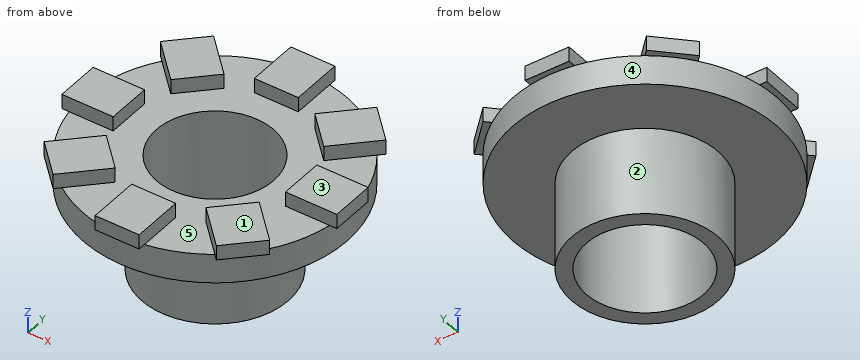
```python
from build123d import *

# Parameters (mm, degrees)
F4_DEPTH = 6.35
F5_COUNT = 8


# Not quite as in the source:
# - a feature names something its author has since deleted; it is built from what else it names


with BuildPart() as f1:
    # F0 (on Front) → F1 (revolve)
    with BuildSketch(Plane.XZ):
        Polygon((25.4, 0), (25.4, -50.8), (31.75, -50.8), (31.75, -12.7), (57.15, -12.7), (57.15, 0), align=None)
    revolve(axis=Axis((0, 0, 2.673143521), (0, 0, -1)))

    # F2 (on face) → F4 (join)
    with BuildSketch(Plane.XY):
        with BuildLine():
            ThreePointArc((57.15, 0), (56.9498143774, -4.779240775), (56.350659934, -9.525))
            Line((56.350659934, -9.525), (59.525659934, -9.525))
            Line((59.525659934, -9.525), (59.525659934, 9.525))
            Line((59.525659934, 9.525), (56.350659934, 9.525))
            ThreePointArc((56.350659934, 9.525), (56.9498143774, 4.779240775), (57.15, 0))
        make_face()
        with BuildLine():
            Line((37.300659934, 9.525), (37.300659934, -9.525))
            Line((37.300659934, -9.525), (56.350659934, -9.525))
            ThreePointArc((56.350659934, -9.525), (56.9498143774, -4.779240775), (57.15, 0))
            ThreePointArc((57.15, 0), (56.9498143774, 4.779240775), (56.350659934, 9.525))
            Line((56.350659934, 9.525), (37.300659934, 9.525))
        make_face()
    extrude(amount=F4_DEPTH)

    # F5: F1 ×8 about axis
    f5_axis = Axis((0, 0, 22.2758), (0, 0, 1))


with BuildPart() as f1_1:
    add(f1.part)
    for i in range(1, F5_COUNT):
        add(f1.part.rotate(f5_axis, i * 360 / F5_COUNT))


solid = f1_1.part
```
Work out the finished part from the listing and answer in its coordinate system (mm). Face numbers are marked on the shaded views. A direction names the side the tool comes from. Round coordinates to 2 decimals unless told otherwise and drop trailing zeros. Loops run counter-clockwise (first coordinate to the right, second up) from the corner with the lowest first, then second, coordinate; pieces in that order, holes last.
(1) The part is cut by section D-D, the plane x = -28.5. Give the vertices of the cut face in (y, z).
Computed values:
outline: (-49.54, -12.7) - (-13.99, -12.7) - (-13.99, -50.8) - (13.99, -50.8) - (13.99, -12.7) - (49.54, -12.7) - (49.54, 0) - (41.97, 0) - (41.97, 6.35) - (24.25, 6.35) - (24.25, 0) - (-24.25, 0) - (-24.25, 6.35) - (-41.97, 6.35) - (-41.97, 0) - (-49.54, 0) - close
(2) For the marked faces 1 and 2, determine the directions among +Z, -Z, +X, -X, +Y, -Y from which every point of the face is accessible in a straight line to the end or side of a thin tool.
Computed values:
face 1: +Z, +X, -X, +Y, -Y
face 2: -Z
(3) Find the intervals of material crossed by L1, parallel to Y at x = 0, z = -39; L2, parallel to Z at x = 41, y = 28, in increasing order.
Computed values:
L1: y = -31.75 to -25.4, 25.4 to 31.75
L2: z = -12.7 to 6.35
(4) The part is cut by section A-A, the plane x = 0. Give the vertices of the cut face in (y, z), and give its area (3 significant figures).
Computed values:
outline: (-59.53, 0) - (-57.15, 0) - (-57.15, -12.7) - (-31.75, -12.7) - (-31.75, -50.8) - (-25.4, -50.8) - (-25.4, 0) - (-37.3, 0) - (-37.3, 6.35) - (-59.53, 6.35) - close; (25.4, -50.8) - (31.75, -50.8) - (31.75, -12.7) - (57.15, -12.7) - (57.15, 0) - (59.53, 0) - (59.53, 6.35) - (37.3, 6.35) - (37.3, 0) - (25.4, 0) - close
area: 1,570 mm2
(5) Each of these flat-tipped pins is pushed along its axis until it touches: P1, Ø4, axis at y = 19.5, z = -12.5, coming from the -X side; P2, Ø1.6, axis at x = 58.5, y = -2, coming from the -Z side; P3, Ø7, axis at x = -54, z = 4.5, coming from the +Y side (3 decimals); P4, Ø6, axis at y = 47, z = -18.5, coming from the +X side. Where does it stop, or does it pass through?
Computed values:
P1: stops at x = -54.4
P2: stops at z = 0
P3: stops at y = 9.525
P4: passes through
(6) The mould has two halves that part along X. Classify the marked faces 3, 4 and 5: pulls with the +X half, pulls with the -X half, needs draft (parallel to the pull), parting line crosses it, or undercut.
Computed values:
face 3: needs draft
face 4: parting line crosses it
face 5: undercut
(7) The part is cut by section C-C, the plane z = -17.5. Give the vertices of the cut face in (x, y), and give its area (3 significant figures).
Computed values:
outline: circle Ø63.5 at (0, 0); hole circle Ø50.8 at (0, 0)
area: 1,140 mm2
